Can you work these out from the model? Positions are in its coordinate system, mm. A direction names the side the tool comes from. Give positions to 0.01 mm unless a question says otherwise; leave off trailing zeros. Order: outer loops, then holes, each group sorted by start corner. A loop starts at its lowest first (then second) coordinate and runs counter-clockwise, first axis right, second up. Notation, with made-up numbers: (62, 13.5) -> (80, 13.5) arc R23 cw to (80, 24.5) -> close; hole circle Ø11 at (89, 66.5). An arc over 180 degrees is marked (long way). Answer as a JSON object with one key per item and string values.
```python
from build123d import *

# Parameters (mm, degrees)
REDONDEO1_R           = 0.2
CHAFL_N1_SIZE         = 0.5
CORTAR_EXTRUIR1_DEPTH = 2.75


with BuildPart() as part:
    # Croquis1 → Revolución1 (revolve)
    with BuildSketch(Plane(origin=(0, 0, 0), x_dir=(0, 0, -1), z_dir=(1, 0, 0))):
        Polygon((0, 3), (3.63504566, 3), (3.63504566, 2.862019845), (4, 2.862019845), (4, 1.955), (18, 1.955), (18, 0), (0, 0), align=None)
    revolve(axis=Axis((0, 0, -18), (0, 0, 1)))

    # Redondeo1
    redondeo1_edges = [part.edges().sort_by_distance(p)[0] for p in [
        (0, -1.955, -4),
    ]]
    fillet(redondeo1_edges, radius=REDONDEO1_R)

    # Chaflán1
    chafl_n1_edges = [part.edges().sort_by_distance(p)[0] for p in [
        (0, -1.955, -18),
    ]]
    chamfer(chafl_n1_edges, length=CHAFL_N1_SIZE)

    # Croquis2 → Cortar-Extruir1 (cut)
    with BuildSketch(Plane.XY):
        Polygon((-1.625, 0), (-0.8125, -1.407291281), (0.8125, -1.407291281), (1.625, 0), (0.8125, 1.407291281), (-0.8125, 1.407291281), align=None)
    extrude(amount=-CORTAR_EXTRUIR1_DEPTH, mode=Mode.SUBTRACT)


solid = part.part
```
1. Please list where these lines run through material, in increasing order: L1, parallel to Z at x = 0.5, y = 2.45; L2, parallel to Z at x = -1.15, y = 0.35; L3, parallel to Y at x = 0.1, z = -4.5.
Worked answers:
{"L1": "-4 to 0", "L2": "-18 to -2.75", "L3": "-1.95 to 1.95"}
2. If we mould it in two halves opening along Y, with no side actions, what happens to faces 1 (the face through (0, 0, -18)), 2 (the face through (1.213, -0.713, -1.356)), 3 (the face through (-0.587, 1.865, -10.943))? For each: +Y half, -Y half, draft (parallel to the pull), parting line (faces both ways), or undercut.
Worked answers:
{"face 1": "draft", "face 2": "undercut", "face 3": "parting line"}
3. If we section it at A-A on x = 0: Please give me the cut outline in (y, z) (3 decimals), then the cut area to 3 significant figures.
Worked answers:
{"outline": "(-3, -3.635) -> (-2.862, -3.635) -> (-2.862, -4) -> (-2.155, -4) arc R0.2 cw to (-1.955, -4.2) -> (-1.955, -17.5) -> (-1.455, -18) -> (1.455, -18) -> (1.955, -17.5) -> (1.955, -4.2) arc R0.2 cw to (2.155, -4) -> (2.862, -4) -> (2.862, -3.635) -> (3, -3.635) -> (3, 0) -> (1.407, 0) -> (1.407, -2.75) -> (-1.407, -2.75) -> (-1.407, 0) -> (-3, 0) -> close", "area": "70.7 mm²"}
4. Will these pins go through, and if not, where does the flat tip stop? pin 1 Ø1 at (y, z) = (-2, -5.5) entering from +X; pin 2 Ø1.4 at (x, y) = (0, 0) entering from +Z.
Worked answers:
{"pin 1": "x = 1.25", "pin 2": "z = -2.75"}
5. If we section it at B-B on z = -15: Please give me the cut outline in (x, y) (3 decimals), then the cut area to 3 significant figures.
Worked answers:
{"outline": "circle Ø3.91 at (0, 0)", "area": "12.0 mm²"}
6. For faces 4 (the face through (-2.413, 1.539, -3.82)), 5 (the face through (-1.224, -0.694, -1.356)), 6 (the face through (-1.4, 0.7, 0)), which set-ups out of +Z, -Z, +X, -X, +Y, -Y let a thin tool reach every point of the face, with its end or its side?
Worked answers:
{"face 4": "-Z", "face 5": "+Z", "face 6": "+Z, +X, -X, +Y, -Y"}
7. If we section it at C-C on x = 2.65: Please give me the cut outline in (y, z), then the cut area to 3 significant figures.
Worked answers:
{"outline": "(-1.41, -3.64) -> (-1.08, -3.64) -> (-1.08, -4) -> (1.08, -4) -> (1.08, -3.64) -> (1.41, -3.64) -> (1.41, 0) -> (-1.41, 0) -> close", "area": "11.0 mm²"}
